Geometry: final body of the model. Coordinates: model frame, mm. Coordinates: 2 decimals unless noted, no trailing zeros. Loops run counter-clockwise (first coordinate to the right, second up) from the corner with the lowest first, then second, coordinate; pieces in that order, holes last. Notation, with made-up numbers: (-20, 4.5) -> (-3, 4.5) arc R17 cw to (-3, 22.5) -> close; hole circle Ø6 at (66, 36). An arc over 180 degrees is marked (long way). One line per item, written item: value. Start each with the question number.
Item 1: Section query C-C on x = 28. Return loops of the section in (y, z), then the cut area to 3 significant figures.
Item 2: Section query A-A on z = 101.5. Return loops of the section in (x, y), then the cut area to 3 significant figures.
Item 3: Ray query, probe 1 along X at (y, z) = (-0.85, 0); probe 2 along Z at (x, y) = (-0.5, -2.5); probe 3 along Z at (x, y) = (-5, -2.25). Return the intervals inside material, ascending. Write a range as from..to.
Item 4: Section query D-D on z = 45. Return loops of the section in (x, y).
Item 5: Section query B-B on y = -1.65. Give the number of separate pieces and of enclosed holes in the cut face, then the cut area to 3 significant figures.
Item 6: Contact query for flat-ended pins moving along their axis: pin 1 Ø1 at (y, z) = (-1.5, 62) entering from -X; pin 2 Ø1 at (x, y) = (7, -2.5) entering from +Z; pin 3 Ø1 at (y, z) = (-2.5, 95) entering from +X. Output: stop coordinate, or through.
from build123d import *

# Parameters (mm, degrees)
F0_R     = 3.175
F1_DEPTH = 3.048


with BuildPart() as f1:
    # F0 (on Front) → F1 (new body)
    with BuildSketch(Plane.XZ):
        with BuildLine():
            ThreePointArc((1.5875, 0), (-1.1225320151, -1.1225320151), (0, 1.5875))
            Line((0, 1.5875), (0, 9.525))
            ThreePointArc((0, 9.525), (-7.063929059, 6.3895642457), (-9.4772553384, -0.9525))
            ThreePointArc((-9.4772553384, -0.9525), (-6.3895642457, -7.063929059), (0, -9.525))
            Line((0, -9.525), (0.6773435479, -9.500885786))
            ThreePointArc((0.6773435479, -9.500885786), (6.9705567315, -6.4912990883), (9.525, 0))
            Line((9.525, 0), (1.5875, 0))
        make_face()
        with BuildLine():
            ThreePointArc((-9.4772553384, -0.9525), (-7.063929059, 6.3895642457), (0, 9.525))
            Line((0, 9.525), (0, 47.625))
            ThreePointArc((0, 47.625), (-10.6492737428, 51.7267849017), (-15.7954255641, 61.9125))
            Line((-15.7954255641, 61.9125), (-9.4772553384, -0.9525))
        make_face()
        with BuildLine():
            Line((0, 47.625), (0, 9.525))
            ThreePointArc((0, 9.525), (6.7351920908, 6.7351920908), (9.525, 0))
            Line((9.525, 0), (36.5125, 0))
            ThreePointArc((36.5125, 0), (38.8373399243, 5.6126600757), (44.45, 7.9375))
            Line((44.45, 7.9375), (19.0516679685, 7.9375))
            ThreePointArc((19.0516679685, 7.9375), (13.1719464369, 10.5365735064), (11.1366133377, 16.6344196472))
            Line((11.1366133377, 16.6344196472), (15.0940259351, 58.5820729906))
            ThreePointArc((15.0940259351, 58.5820729906), (9.3258654753, 50.6530603591), (0, 47.625))
        make_face()
        with BuildLine():
            Line((36.5125, 0), (9.525, 0))
            ThreePointArc((9.525, 0), (6.9705567315, -6.4912990883), (0.6773435479, -9.500885786))
            Line((0.6773435479, -9.500885786), (44.7324052746, -7.9324746146))
            ThreePointArc((44.7324052746, -7.9324746146), (38.9380895153, -5.7116327839), (36.5125, 0))
        make_face()
        with BuildLine():
            ThreePointArc((-15.7954255641, 61.9125), (-10.6492737428, 51.7267849017), (0, 47.625))
            Line((0, 47.625), (0, 61.9125))
            ThreePointArc((0, 61.9125), (-1.5875, 63.5), (0, 65.0875))
            Line((0, 65.0875), (0, 79.375))
            ThreePointArc((0, 79.375), (-10.4912828548, 75.4142187767), (-15.7474569047, 65.5082893304))
            ThreePointArc((-15.7474569047, 65.5082893304), (-15.8735876171, 63.7117573215), (-15.7954255641, 61.9125))
        make_face()
        with BuildLine():
            Line((0, 61.9125), (0, 47.625))
            ThreePointArc((0, 47.625), (9.3258654753, 50.6530603591), (15.0940259351, 58.5820729906))
            Line((15.0940259351, 58.5820729906), (15.7474569047, 65.5082893304))
            ThreePointArc((15.7474569047, 65.5082893304), (10.4912828548, 75.4142187767), (0, 79.375))
            Line((0, 79.375), (0, 65.0875))
            ThreePointArc((0, 65.0875), (1.1225320151, 64.6225320151), (1.5875, 63.5))
            ThreePointArc((1.5875, 63.5), (1.1225320151, 62.3774679849), (0, 61.9125))
        make_face()
        with BuildLine():
            ThreePointArc((44.45, 7.9375), (38.8373399243, 5.6126600757), (36.5125, 0))
            ThreePointArc((36.5125, 0), (38.9380895153, -5.7116327839), (44.7324052746, -7.9324746146))
            ThreePointArc((44.7324052746, -7.9324746146), (50.1616327839, -5.5119104847), (52.3875, 0))
            ThreePointArc((52.3875, 0), (50.0626600757, 5.6126600757), (44.45, 7.9375))
        make_face()
        with BuildLine():
            ThreePointArc((46.0375, 0), (44.45, -1.5875), (42.8625, 0))
            ThreePointArc((42.8625, 0), (44.45, 1.5875), (46.0375, 0))
        make_face(mode=Mode.SUBTRACT)
        with BuildLine():
            ThreePointArc((0, -9.525), (0.3388863295, -9.5189695375), (0.6773435479, -9.500885786))
            Line((0.6773435479, -9.500885786), (0, -9.525))
        make_face()
        with BuildLine():
            Line((15.7474569047, 65.5082893304), (15.0940259351, 58.5820729906))
            ThreePointArc((15.0940259351, 58.5820729906), (15.6785408556, 61.0102245804), (15.875, 63.5))
            ThreePointArc((15.875, 63.5), (15.8430821396, 64.5061676396), (15.7474569047, 65.5082893304))
        make_face()
        with BuildLine():
            Line((-9.525, 114.3), (-15.7474569047, 65.5082893304))
            ThreePointArc((-15.7474569047, 65.5082893304), (-10.4912828548, 75.4142187767), (0, 79.375))
            Line((0, 79.375), (0, 100.0252))
            Line((0, 100.0252), (0, 104.775))
            ThreePointArc((0, 104.775), (-6.7351920908, 107.5648079092), (-9.525, 114.3))
        make_face()
        with Locations((-3.175, 100.0252)):
            Circle(F0_R, mode=Mode.SUBTRACT)
        with BuildLine():
            ThreePointArc((0, 79.375), (10.4912828548, 75.4142187767), (15.7474569047, 65.5082893304))
            Line((15.7474569047, 65.5082893304), (9.525, 114.3))
            ThreePointArc((9.525, 114.3), (6.7351920908, 107.5648079092), (0, 104.775))
            Line((0, 104.775), (0, 100.0252))
            Line((0, 100.0252), (0, 79.375))
        make_face()
        with BuildLine():
            ThreePointArc((9.525, 114.3), (0, 123.825), (-9.525, 114.3))
            ThreePointArc((-9.525, 114.3), (-6.7351920908, 107.5648079092), (0, 104.775))
            ThreePointArc((0, 104.775), (6.7351920908, 107.5648079092), (9.525, 114.3))
        make_face()
        with BuildLine():
            ThreePointArc((1.5875, 114.3), (1.1225320151, 113.1774679849), (0, 112.7125))
            ThreePointArc((0, 112.7125), (-1.1225320151, 115.4225320151), (1.5875, 114.3))
        make_face(mode=Mode.SUBTRACT)
        with BuildLine():
            Line((0, 9.525), (0, 1.5875))
            ThreePointArc((0, 1.5875), (1.1225320151, 1.1225320151), (1.5875, 0))
            Line((1.5875, 0), (9.525, 0))
            ThreePointArc((9.525, 0), (6.7351920908, 6.7351920908), (0, 9.525))
        make_face()
    extrude(amount=F1_DEPTH)


solid = f1.part
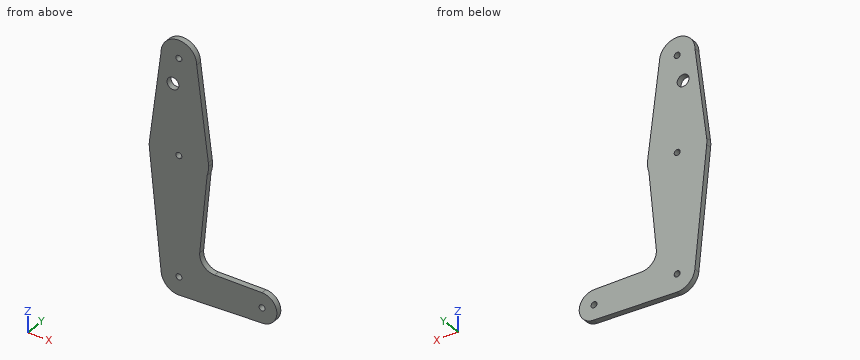
Reply:
1. outline: (-3.05, -8.53) -> (0, -8.53) -> (0, 7.94) -> (-3.05, 7.94) -> close
1. area: 50.2 mm²
2. outline: (-11.16, -3.05) -> (-5.99, -3.05) -> (-5.99, 0) -> (-11.16, 0) -> close; (-0.36, -3.05) -> (11.16, -3.05) -> (11.16, 0) -> (-0.36, 0) -> close
2. area: 50.9 mm²
3. probe 1: x = -9.57..-1.59, 1.59..42.86, 46.04..52.39
3. probe 2: z = -9.51..-1.51, 1.51..61.99, 65.01..98.31, 101.74..112.79, 115.81..123.81
3. probe 3: z = -8.11..97.43, 102.62..122.41
4. outline: (-14.1, -3.05) -> (13.81, -3.05) -> (13.81, 0) -> (-14.1, 0) -> close
5. separate pieces: 1
5. enclosed holes: 5
5. area: 3,830 mm²
6. pin 1: stops at x = -15.84
6. pin 2: stops at z = 121.26
6. pin 3: stops at x = 12.05
